The listing builds one solid part. Answer for the finished solid, in the listing's coordinates (mm). Round coordinates to 2 decimals unless told otherwise and drop trailing zeros. Write each loop counter-clockwise with the first axis right and the second up, starting at its lowest first coordinate (ties: lowest second). Pieces come first, ordered by that corner, then holes.
Item 1: Find the intervals of material crossed by probe 1 along Y at (x, z) = (7.25, 4.9); probe 2 along X at (y, z) = (-4, 4); probe 3 along Z at (x, y) = (6.5, -7), in increasing order.
Item 2: Each of these flat-tipped pins is pushed along its axis until it touches: pin 1 (1 mm diameter, centred on y = -3, z = 4.5, fed in from -X); pin 2 (1 mm diameter, centred on x = 4.5, y = -1, fed in from -Z); pin 3 (1 mm diameter, centred on y = -7.5, z = 4, fed in from +X). Where does it stop, or does it pass through?
Item 3: Find section A-A on y = -2. Give the vertices of the cut face in (x, z), then the cut area to 3 significant figures.
Item 4: For a pull along X with two mould halves and no side action, classify faces 1 (the face through (8.563, -3.73, 2.774)), 2 (the face through (5, -8.9, 2)), 3 (the face through (5, -4, 0.4)) as +X half, -X half, draft (parallel to the pull), parting line (faces both ways), or undercut.
Item 5: Find section B-B on x = 6. Give the vertices of the cut face in (y, z), then the cut area to 3 significant figures.
Item 6: Find section C-C on x = 3.5. Give the vertices of the cut face in (y, z), then the cut area to 3 significant figures.
```python
from build123d import *

# Parameters (mm, degrees)
BOX019_W           = 8.5
BOX019_H           = 14
BOX019_DEPTH       = 0.5
CHAMFER_SIZE       = 0.45
BOX014_W           = 8.7
BOX014_H           = 10.2
BOX014_DEPTH       = 6.15
BOX014_PITCH_ANGLE = 60
BOX013_W           = 8.7
BOX013_H           = 12.2
BOX013_DEPTH       = 11.15
BOX013_PITCH_ANGLE = 60
BOX012_W           = 8.7
BOX012_H           = 10.2
BOX012_DEPTH       = 6.15
BOX012_PITCH_ANGLE = 60
BOX011_W           = 11
BOX011_H           = 10.2
BOX011_DEPTH       = 6.15
FILLET002_R        = 0.1
FILLET003_R        = 0.1


with BuildPart() as chamfer_body:
    # Box019 → Box019 (new body)
    with BuildSketch(Plane(origin=(1, -11, -0.1), x_dir=(1, 0, 0), z_dir=(0, 0, 1))):
        with Locations((4.25, 7)):
            Rectangle(BOX019_W, BOX019_H)
    extrude(amount=BOX019_DEPTH)

    # Chamfer
    chamfer_edges = [chamfer_body.edges().sort_by_distance(p)[0] for p in [
        (9.5, -4, 0.4),
    ]]
    chamfer(chamfer_edges, length=CHAMFER_SIZE)


with BuildPart() as kub014:
    # Box014 → Box014 (new body)
    with BuildSketch(Plane.XY):
        with Locations((4.35, 5.1)):
            Rectangle(BOX014_W, BOX014_H)
    extrude(amount=BOX014_DEPTH)


with BuildPart() as kub014_1:
    # Box014 pitch: moved
    add(kub014.part.rotate(Axis((0, 0, 0), (0, 1, 0)), BOX014_PITCH_ANGLE))


with BuildPart() as kub014_2:
    # Box014 placement: moved
    add(kub014_1.part.moved(Location((-7.8, -8.9, 2))))


with BuildPart() as kub013:
    # Box013 → Box013 (new body)
    with BuildSketch(Plane.XY):
        with Locations((4.35, 6.1)):
            Rectangle(BOX013_W, BOX013_H)
    extrude(amount=BOX013_DEPTH)


with BuildPart() as kub013_1:
    # Box013 pitch: moved
    add(kub013.part.rotate(Axis((0, 0, 0), (0, 1, 0)), BOX013_PITCH_ANGLE))


with BuildPart() as kub013_2:
    # Box013 placement: moved
    add(kub013_1.part.moved(Location((-5.72, -9.9, 8.17))))


with BuildPart() as kub012:
    # Box012 → Box012 (new body)
    with BuildSketch(Plane.XY):
        with Locations((4.35, 5.1)):
            Rectangle(BOX012_W, BOX012_H)
    extrude(amount=BOX012_DEPTH)


with BuildPart() as kub012_1:
    # Box012 pitch: moved
    add(kub012.part.rotate(Axis((0, 0, 0), (0, 1, 0)), BOX012_PITCH_ANGLE))


with BuildPart() as kub012_2:
    # Box012 placement: moved
    add(kub012_1.part.moved(Location((6.7, -8.9, 6))))


with BuildPart() as fillet003:
    # Box011 → Box011 (new body)
    with BuildSketch(Plane(origin=(-0.5, -8.9, 0), x_dir=(1, 0, 0), z_dir=(0, 0, 1))):
        with Locations((5.5, 5.1)):
            Rectangle(BOX011_W, BOX011_H)
    extrude(amount=BOX011_DEPTH)

    # Cut007: cut Kub012
    add(kub012_2.part, mode=Mode.SUBTRACT)

    # Cut008: cut Kub013
    add(kub013_2.part, mode=Mode.SUBTRACT)

    # Cut009: cut Kub014
    add(kub014_2.part, mode=Mode.SUBTRACT)

    # Cut010: cut Chamfer body
    add(chamfer_body.part, mode=Mode.SUBTRACT)

    # Fillet002
    fillet002_edges = [fillet003.edges().sort_by_distance(p)[0] for p in [
        (1, -8.9, 0.2),
        (5.025, -8.9, 0.4),
        (9.25, -8.9, 0.2),
    ]]
    fillet(fillet002_edges, radius=FILLET002_R)

    # Fillet003
    fillet003_edges = [fillet003.edges().sort_by_distance(p)[0] for p in [
        (8.584732, -8.9, 2.735548),
        (8.584732, 1.3, 2.735548),
        (1, 1.3, 0.2),
        (5.025, 1.3, 0.4),
        (9.25, 1.3, 0.2),
    ]]
    fillet(fillet003_edges, radius=FILLET003_R)


solid = fillet003.part
```
Check values:
1. probe 1: y = -8.9 to 1.3
1. probe 2: x = 4.46 to 7.85
1. probe 3: z = 0.4 to 5.18
2. pin 1: stops at x = 4.46
2. pin 2: stops at z = 0.4
2. pin 3: stops at x = 8.14
3. outline: (-0.28, 1.27) - (0.46, 0) - (1, 0) - (1, 0.4) - (9.05, 0.4) - (9.45, 0) - (10.16, 0) - (7.01, 5.47) - close
3. area: 29.4 mm2
4. face 1: +X half
4. face 2: draft
4. face 3: undercut
5. outline: (-8.9, 0.5) arc R0.1 ccw to (-8.8, 0.4) - (1.2, 0.4) arc R0.1 ccw to (1.3, 0.5) - (1.3, 4.89) - (-8.9, 4.89) - close
5. area: 45.8 mm2
6. outline: (-8.9, 0.5) arc R0.1 ccw to (-8.8, 0.4) - (1.2, 0.4) arc R0.1 ccw to (1.3, 0.5) - (1.3, 3.45) - (-8.9, 3.45) - close
6. area: 31.1 mm2
